```python
from build123d import *

# Parameters (mm, degrees)
ESQUISSE1_R        = 1.75
ESQUISSE1_R_2      = 10
ESQUISSE1_R_3      = 5.125
ESQUISSE1_R_4      = 4
BOSS_EXTRU_1_DEPTH = 6


with BuildPart() as part:
    # Esquisse1 → Boss.-Extru.1 (new body)
    with BuildSketch(Plane.XY):
        with BuildLine():
            Line((-94, -75), (-94, 75))
            ThreePointArc((-94, 75), (-91.071067812, 82.071067812), (-84, 85))
            Line((-84, 85), (84, 85))
            ThreePointArc((84, 85), (91.071067812, 82.071067812), (94, 75))
            Line((94, 75), (94, -75))
            ThreePointArc((94, -75), (91.071067812, -82.071067812), (84, -85))
            Line((84, -85), (-84, -85))
            ThreePointArc((-84, -85), (-91.071067812, -82.071067812), (-94, -75))
        make_face()
        with Locations((-84, 75)):
            Circle(ESQUISSE1_R, mode=Mode.SUBTRACT)
        with Locations((84, 75)):
            Circle(ESQUISSE1_R, mode=Mode.SUBTRACT)
        with Locations((84, -75)):
            Circle(ESQUISSE1_R, mode=Mode.SUBTRACT)
        with Locations((-84, -75)):
            Circle(ESQUISSE1_R, mode=Mode.SUBTRACT)
        with Locations((-82, -35.7)):
            Circle(ESQUISSE1_R, mode=Mode.SUBTRACT)
        with Locations((-82, -10.5)):
            Circle(ESQUISSE1_R, mode=Mode.SUBTRACT)
        with Locations((-82, 14.7)):
            Circle(ESQUISSE1_R, mode=Mode.SUBTRACT)
        with Locations((-16, -35.7)):
            Circle(ESQUISSE1_R, mode=Mode.SUBTRACT)
        with Locations((-3.5, -23.5)):
            Circle(ESQUISSE1_R, mode=Mode.SUBTRACT)
        with Locations((86.5, -23.5)):
            Circle(ESQUISSE1_R, mode=Mode.SUBTRACT)
        with Locations((86.5, -2.625)):
            Circle(ESQUISSE1_R, mode=Mode.SUBTRACT)
        with Locations((86.5, 18.25)):
            Circle(ESQUISSE1_R, mode=Mode.SUBTRACT)
        with Locations((86.5, 39.125)):
            Circle(ESQUISSE1_R, mode=Mode.SUBTRACT)
        with Locations((-3.5, -2.625)):
            Circle(ESQUISSE1_R, mode=Mode.SUBTRACT)
        with Locations((-3.5, 39.125)):
            Circle(ESQUISSE1_R, mode=Mode.SUBTRACT)
        with Locations((-16, -10.5)):
            Circle(ESQUISSE1_R, mode=Mode.SUBTRACT)
        with Locations((-16, 14.7)):
            Circle(ESQUISSE1_R, mode=Mode.SUBTRACT)
        with Locations((-58, -70.9)):
            Circle(ESQUISSE1_R, mode=Mode.SUBTRACT)
        with Locations((-40, -70.9)):
            Circle(ESQUISSE1_R, mode=Mode.SUBTRACT)
        with Locations((55, -70.9)):
            Circle(ESQUISSE1_R, mode=Mode.SUBTRACT)
        with Locations((-35, 35)):
            Circle(ESQUISSE1_R, mode=Mode.SUBTRACT)
        with Locations((35, 35)):
            Circle(ESQUISSE1_R, mode=Mode.SUBTRACT)
        with Locations((35, -35)):
            Circle(ESQUISSE1_R, mode=Mode.SUBTRACT)
        with Locations((-35, -35)):
            Circle(ESQUISSE1_R, mode=Mode.SUBTRACT)
        with Locations((0, -70.9)):
            Circle(ESQUISSE1_R_2, mode=Mode.SUBTRACT)
        with Locations((84, 57.0625)):
            Circle(ESQUISSE1_R_3, mode=Mode.SUBTRACT)
        with Locations((69.210172414, -75)):
            Circle(ESQUISSE1_R_4, mode=Mode.SUBTRACT)
        with BuildLine():
            Line((-9.75, 78.928270362), (-9.75, 82.928270362))
            Line((-9.75, 82.928270362), (-7.25, 82.928270362))
            Line((-7.25, 82.928270362), (-7.25, 78.928270362))
            ThreePointArc((-7.25, 78.928270362), (-8.5, 62.775), (-9.75, 78.928270362))
        make_face(mode=Mode.SUBTRACT)
    extrude(amount=BOSS_EXTRU_1_DEPTH)


solid = part.part
```
Work out the finished part from the listing and answer in its coordinate system (mm). A direction names the side the tool comes from. Coordinates: 2 decimals unless noted, no trailing zeros. Write each loop counter-clockwise with the first axis right and the second up, starting at its lowest first coordinate (ties: lowest second). Pieces come first, ordered by that corner, then holes. Notation, with made-up numbers: (5.25, 26.25) - (25.25, 26.25) arc R12 ccw to (25.25, 45.25) - close; hole circle Ø3 at (48.5, -1). An arc over 180 degrees is marked (long way). Answer as a JSON object with one key per item and string values.
Q1. For a pull along Y with two mould halves and no side action, classify faces 1 (the cylindrical face through (91.15, -81.99, 2.96)), 2 (the flat face through (-1, 85, 3)), 3 (the flat face through (-7.25, 81, 3)) as pulls with the +Y half, pulls with the -Y half, needs draft (parallel to the pull), parting line crosses it, or undercut.
Results list:
{"face 1": "pulls with the -Y half", "face 2": "pulls with the +Y half", "face 3": "undercut"}
Q2. Find section C-C (z = 4). State how many separate pieces and enclosed holes the cut face has, plus the area to 3 significant figures.
Results list:
{"separate pieces": "1", "enclosed holes": "28", "area": "31,000 mm^2"}
Q3. Which of the six approach directions +Z, -Z, +X, -X, +Y, -Y give full straight-line access (tool end or side, diameter ignored) to faces 4 (the flat face through (-9.75, 81, 3)), 5 (the cylindrical face through (-90.99, -82.15, 2.96))?
Results list:
{"face 4": "+Z, -Z", "face 5": "+Z, -Z, -X, -Y"}
Q4. Find section B-B (x = 7). Write down the section's boundary in (y, z), plus the area to 3 significant figures.
Results list:
{"outline": "(-85, 0) - (-78.04, 0) - (-78.04, 6) - (-85, 6) - close; (-63.76, 0) - (85, 0) - (85, 6) - (-63.76, 6) - close", "area": "934 mm^2"}
Q5. Find section A-A (y = 70.9). Write down the section's boundary in (x, z) (3 decimals), plus the area to 3 significant figures.
Results list:
{"outline": "(-94, 0) - (-16.625, 0) - (-16.625, 6) - (-94, 6) - close; (-0.375, 0) - (94, 0) - (94, 6) - (-0.375, 6) - close", "area": "1,030 mm^2"}
Q6. Given pin 1 Ø5.5 at (x, y) = (55, -70.9) entering from +Z; pin 2 Ø2 at (y, z) = (80.5, 3) entering from +X, each flat-ended and moving along its own axis, determine where each tip first touches the part or whether it passes through.
Results list:
{"pin 1": "stops at z = 6", "pin 2": "stops at x = 92.93"}
Q7. Consider L1, parallel to Y at x = 84, z = 2.35; L2, parallel to X at y = -70.5, z = 3.2; L3, parallel to Y at x = 0, z = 2.25. Determine where each line is inside the solid, lowest interval first. Write a range as from..to.
Results list:
{"L1": "y = -85..-76.75, -73.25..51.94, 62.19..73.25, 76.75..85", "L2": "x = -94..-59.7, -56.3..-41.7, -38.3..-9.99, 9.99..53.3, 56.7..94", "L3": "y = -85..-80.9, -60.9..85"}
